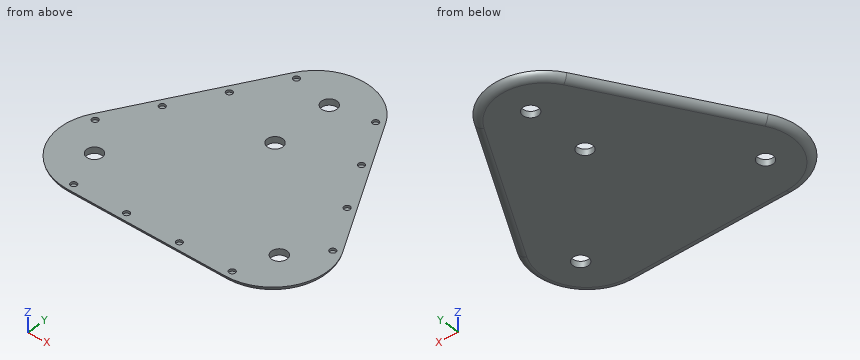
```python
from build123d import *

# Parameters (mm, degrees)
RESSALTO_EXTRUS_O1_DEPTH = 4
ESBO_O2_R                = 5
CORTE_EXTRUS_O1_DEPTH    = 4
ESBO_O3_R                = 2.025
CORTE_EXTRUS_O2_DEPTH    = 1.5
FILETE1_R                = 5


with BuildPart() as part:
    # Esboço1 → Ressalto-extrusão1 (new body)
    with BuildSketch(Plane.XY):
        with BuildLine():
            Line((-30.310889132, 77.5), (-82.27241336, -12.5))
            ThreePointArc((-82.27241336, -12.5), (-82.27241336, -47.5), (-51.961524227, -65))
            Line((-51.961524227, -65), (51.961524227, -65))
            ThreePointArc((51.961524227, -65), (82.27241336, -47.5), (82.27241336, -12.5))
            Line((82.27241336, -12.5), (30.310889132, 77.5))
            ThreePointArc((30.310889132, 77.5), (0, 95), (-30.310889132, 77.5))
        make_face()
    extrude(amount=RESSALTO_EXTRUS_O1_DEPTH)

    # Esboço2 → Corte-extrusão1 (cut)
    with BuildSketch(Plane.XY):
        with Locations((0, 70)):
            Circle(ESBO_O2_R)
        with Locations((60.621778265, -35)):
            Circle(ESBO_O2_R)
        with Locations((-60.621778265, -35)):
            Circle(ESBO_O2_R)
        with Locations((0, 30)):
            Circle(ESBO_O2_R)
    extrude(amount=CORTE_EXTRUS_O1_DEPTH, mode=Mode.SUBTRACT)

    # Esboço3 → Corte-extrusão2 (cut)
    with BuildSketch(Plane.XY.offset(4)):
        with Locations((-77.942286341, -15)):
            Circle(ESBO_O3_R)
        with Locations((-51.961524227, -60)):
            Circle(ESBO_O3_R)
        with Locations((77.942286341, -15)):
            Circle(ESBO_O3_R)
        with Locations((-60.622286341, 14.999119987)):
            Circle(ESBO_O3_R)
        with Locations((-43.302286341, 44.998239974)):
            Circle(ESBO_O3_R)
        with Locations((-25.982286341, 74.997359961)):
            Circle(ESBO_O3_R)
        with Locations((60.622286341, 14.999119987)):
            Circle(ESBO_O3_R)
        with Locations((43.302286341, 44.998239974)):
            Circle(ESBO_O3_R)
        with Locations((25.982286341, 74.997359961)):
            Circle(ESBO_O3_R)
        with Locations((-17.321524227, -60)):
            Circle(ESBO_O3_R)
        with Locations((17.318475773, -60)):
            Circle(ESBO_O3_R)
        with Locations((51.958475773, -60)):
            Circle(ESBO_O3_R)
    extrude(amount=-CORTE_EXTRUS_O2_DEPTH, mode=Mode.SUBTRACT)

    # Filete1
    # the kernel refuses this fillet: 5 mm, written as the material it takes off along each edge
    with BuildSketch(Plane(origin=(-51.961524227, -30, 0), x_dir=(-0.8660254037844398, 0.49999999999999795, 0), z_dir=(0.49999999999999795, 0.8660254037844398, 0))) as filete1_piece_1:
        with BuildLine():
            CenterArc((30.101020514, 5), FILETE1_R, 270, 78.463040967)
            Line((35, 4), (35.09797959, 3.98))
            ThreePointArc((35.09797959, 3.98), (35.1, 2), (35.1, 0))
            Line((35.1, 0), (35, -0.1))
            Line((35, -0.1), (30.101020514, -0.1))
            Line((30.101020514, -0.1), (30.101020514, 0))
        make_face()
    revolve(axis=Axis((-51.961524227, -30, 0), (0, 0, 1)), revolution_arc=120, mode=Mode.SUBTRACT)
    with BuildSketch(Plane(origin=(-30.310889132, 77.5, 0), x_dir=(0.8660254037844398, -0.4999999999999981, 0), z_dir=(-0.4999999999999981, -0.8660254037844398, 0)), Plane(origin=(-51.961524227, -65, 0), x_dir=(0, 1, 0), z_dir=(1, 0, 0))) as filete1_piece_2:
        with BuildLine():
            CenterArc((4.898979486, 5), FILETE1_R, 191.536959033, 78.463040967)
            Line((0, 4), (-0.09797959, 3.98))
            ThreePointArc((-0.09797959, 3.98), (-0.1, 2), (-0.1, 0))
            Line((-0.1, 0), (0, -0.1))
            Line((0, -0.1), (4.898979486, -0.1))
            Line((4.898979486, -0.1), (4.898979486, 0))
        make_face()
    extrude(amount=103.923048454, mode=Mode.SUBTRACT)
    with BuildSketch(Plane(origin=(0, 60, 0), x_dir=(0.8660254037844363, 0.5000000000000041, 0), z_dir=(0.5000000000000041, -0.8660254037844363, 0))) as filete1_piece_3:
        with BuildLine():
            CenterArc((30.101020514, 5), FILETE1_R, 270, 78.463040967)
            Line((30.101020514, 0), (30.101020514, -0.1))
            Line((30.101020514, -0.1), (35, -0.1))
            Line((35, -0.1), (35.1, 0))
            ThreePointArc((35.1, 0), (35.1, 2), (35.09797959, 3.98))
            Line((35.09797959, 3.98), (35, 4))
        make_face()
    revolve(axis=Axis((0, 60, 0), (0, 0, 1)), revolution_arc=120, mode=Mode.SUBTRACT)
    with BuildSketch(Plane(origin=(82.27241336, -12.5, 0), x_dir=(-1.3637382312526318e-12, -7.873546349178999e-13, 1.0), z_dir=(-0.5000000000000043, 0.8660254037844363, 0))) as filete1_piece_4:
        with BuildLine():
            CenterArc((5, -4.898979486), FILETE1_R, 101.536959033, 78.463040967)
            Line((0, -4.898979486), (-0.1, -4.898979486))
            Line((-0.1, -4.898979486), (-0.1, 0))
            Line((-0.1, 0), (0, 0.1))
            ThreePointArc((0, 0.1), (2, 0.1), (3.98, 0.09797959))
            Line((3.98, 0.09797959), (4, 0))
        make_face()
    extrude(amount=103.923048454, mode=Mode.SUBTRACT)
    with BuildSketch(Plane(origin=(51.961524227, -30, 0), x_dir=(0, -1, 0), z_dir=(-1, 0, 0))) as filete1_piece_5:
        with BuildLine():
            CenterArc((30.101020514, 5), FILETE1_R, 270, 78.463040967)
            Line((30.101020514, 0), (30.101020514, -0.1))
            Line((30.101020514, -0.1), (35, -0.1))
            Line((35, -0.1), (35.1, 0))
            ThreePointArc((35.1, 0), (35.1, 2), (35.09797959, 3.98))
            Line((35.09797959, 3.98), (35, 4))
        make_face()
    revolve(axis=Axis((51.961524227, -30, 0), (0, 0, 1)), revolution_arc=120, mode=Mode.SUBTRACT)


solid = part.part
```
Design review of the part built by this model. Coordinates are the model's own, in mm. Coordinates: 2 decimals unless noted, no trailing zeros. Order: outer loops, then holes, each group sorted by start corner. A loop starts at its lowest first (then second) coordinate and runs counter-clockwise, first axis right, second up.
1) Clearance check with flat-ended pins moving along their axes: pin 1 (3 mm diameter, centred on x = 43.3, y = 45, fed in from +Z); pin 2 (1 mm diameter, centred on x = -18, z = 1.5, fed in from +Y). State where each tip first meets the part, or that it passes through.
2) Take a section at B-B, the plane y = -35. State how many separate pieces and enclosed holes the cut face has, and give its area (3 significant figures).
3) Take a section at A-A, the plane x = 0. Give the boundary of the cut face in (y, z).
4) Wall thickness on line 1 along Y through (x, z) = (53, 3.1); line 2 along Z through (x, y) = (-74, -51); line 3 along Y through (x, z) = (63, 2.15): over which ranges is each line inside the solid? List them lowest first.
Returned:
1. pin 1: stops at z = 2.5
1. pin 2: stops at y = 89.06
2. separate pieces: 3
2. enclosed holes: 0
2. area: 603 mm2
3. outline: (-65, 4) arc R5 ccw to (-60.1, 0) - (25, 0) - (25, 4) - close; (35, 0) - (65, 0) - (65, 4) - (35, 4) - close; (75, 0) - (90.1, 0) arc R5 ccw to (95, 4) - (75, 4) - close
4. line 1: y = -64.71 to -61.74, -58.26 to 37.65
4. line 2: z = 0.01 to 4
4. line 3: y = -62.38 to -39.4, -30.6 to 19.3
